from build123d import *

# Parameters (mm, degrees)
F1_DEPTH = 7


with BuildPart() as f1:
    # F0 (on Top) → F1 (new body)
    with BuildSketch(Plane.XY):
        with BuildLine():
            ThreePointArc((11.013950333, -43.3227563745), (12.2534652904, -46.3520190309), (12.6760278509, -49.5976731181))
            ThreePointArc((12.6760278509, -49.5976731181), (11.5436081746, -54.8347326353), (8.3486797715, -59.1360811692))
            Line((8.3486797715, -59.1360811692), (12.9223209509, -56.5546419063))
            ThreePointArc((12.9223209509, -56.5546419063), (14.2308491604, -53.1849737262), (14.6760278509, -49.5976731181))
            ThreePointArc((14.6760278509, -49.5976731181), (14.1878219864, -45.8438083413), (12.7556852478, -42.3396921772))
            Line((12.7556852478, -42.3396921772), (11.013950333, -43.3227563745))
        make_face()
        with BuildLine():
            ThreePointArc((-4.3802724447, -37.7025104296), (4.3472073452, -37.6903866777), (11.013950333, -43.3227563745))
            Line((11.013950333, -43.3227563745), (12.7556852478, -42.3396921772))
            ThreePointArc((12.7556852478, -42.3396921772), (7.6057300665, -37.0462324185), (0.5297543163, -34.9312095415))
            Line((0.5297543163, -34.9312095415), (-4.3802724447, -37.7025104296))
        make_face()
        with BuildLine():
            Line((12.9223209509, -56.5546419063), (8.3486797715, -59.1360811692))
            ThreePointArc((8.3486797715, -59.1360811692), (-9.7202647257, -57.7338967961), (-7.9198073974, -39.7002829134))
            ThreePointArc((-7.9198073974, -39.7002829134), (-6.2306311682, -38.5586098734), (-4.3802724447, -37.7025104296))
            Line((-4.3802724447, -37.7025104296), (0.5297543163, -34.9312095415))
            ThreePointArc((0.5297543163, -34.9312095415), (-12.7331374397, -56.8951387344), (12.9223209509, -56.5546419063))
        make_face()
        with BuildLine():
            ThreePointArc((0.5297543163, -34.9312095415), (7.6057300665, -37.0462324185), (12.7556852478, -42.3396921772))
            Line((12.7556852478, -42.3396921772), (113.1224855781, 14.3090016955))
            Line((113.1224855781, 14.3090016955), (113.1224855781, 28.618003391))
            Line((113.1224855781, 28.618003391), (0.5297543163, -34.9312095415))
        make_face()
        with BuildLine():
            Line((113.1224855781, 14.3090016955), (12.7556852478, -42.3396921772))
            ThreePointArc((12.7556852478, -42.3396921772), (14.1878219864, -45.8438083413), (14.6760278509, -49.5976731181))
            ThreePointArc((14.6760278509, -49.5976731181), (14.2308491604, -53.1849737262), (12.9223209509, -56.5546419063))
            Line((12.9223209509, -56.5546419063), (113.1224855781, 0))
            Line((113.1224855781, 0), (113.1224855781, 14.3090016955))
        make_face()
    extrude(amount=F1_DEPTH)


solid = f1.part
Geometry: final body of the model. Coordinates: model frame, mm. Give positions to 0.01 mm unless a question says otherwise; leave off trailing zeros. Order: outer loops, then holes, each group sorted by start corner. A loop starts at its lowest first (then second) coordinate and runs counter-clockwise, first axis right, second up. Notation, with made-up numbers: (-17, 17) -> (18, 17) arc R27 cw to (18, 36) -> close; hole circle Ø9 at (-18, 13). An arc over 180 degrees is marked (long way). Answer as a JSON object with one key per item and string values.
Q1. Section C-C (x = 64.5). Output: boundary loops of the cut face in (y, z), plus the area to 3 significant figures.
Entries:
{"outline": "(-27.44, 0) -> (1.17, 0) -> (1.17, 7) -> (-27.44, 7) -> close", "area": "200 mm^2"}
Q2. First-contact query: pin 1 (3 mm diameter, centred on x = 88.5, z = 3.5, fed in from +Y); pin 2 (1 mm diameter, centred on x = 39.5, z = 5.5, fed in from -Y); pin 3 (4 mm diameter, centred on x = 57, z = 6, fed in from +Y). Flat tips, straight axial feed; report the tip coordinate or a pass-through.
Entries:
{"pin 1": "stops at y = 15.57", "pin 2": "stops at y = -41.84", "pin 3": "stops at y = -1.93"}
Q3. Section B-B (z = 5.75). Output: boundary loops of the cut face in (x, y), plus the area to 3 significant figures.
Entries:
{"outline": "(0.53, -34.93) arc R14.68 ccw (long way) to (12.92, -56.55) -> (113.12, 0) -> (113.12, 28.62) -> close; hole circle Ø25.35 at (0, -49.6)", "area": "3,090 mm^2"}
Q4. Section D-D (y = 16.5). Output: boundary loops of the cut face in (x, z), plus the area to 3 significant figures.
Entries:
{"outline": "(91.65, 0) -> (113.12, 0) -> (113.12, 7) -> (91.65, 7) -> close", "area": "150 mm^2"}
Q5. Section A-A (y = -51.5). Output: boundary loops of the cut face in (x, z), plus the area to 3 significant figures.
Entries:
{"outline": "(-14.55, 0) -> (-12.53, 0) -> (-12.53, 7) -> (-14.55, 7) -> close; (12.53, 0) -> (21.88, 0) -> (21.88, 7) -> (12.53, 7) -> close", "area": "79.6 mm^2"}
Q6. Material intervals for probe 1 along X at (y, z) = (-45, 4.25); probe 2 along X at (y, z) = (-39, 6.25); probe 3 along Y at (x, z) = (3.5, 0.75), sorted ascending.
Entries:
{"probe 1": "x = -13.94 to -11.81, 11.81 to 33.39", "probe 2": "x = -10.15 to -6.95, 6.95 to 44.02", "probe 3": "y = -63.85 to -61.78, -37.41 to -33.25"}
Q7. Draft query along Z for faces 1 (the flat face through (58, -18, 7)), 2 (the flat face through (57.614, -2.712, 3.451)), 3 (the flat face through (58, -18, 0)). Return one class per face: released by +Z, released by -Z, zero draft, split by the parting line, or undercut.
Entries:
{"face 1": "released by +Z", "face 2": "zero draft", "face 3": "released by -Z"}
